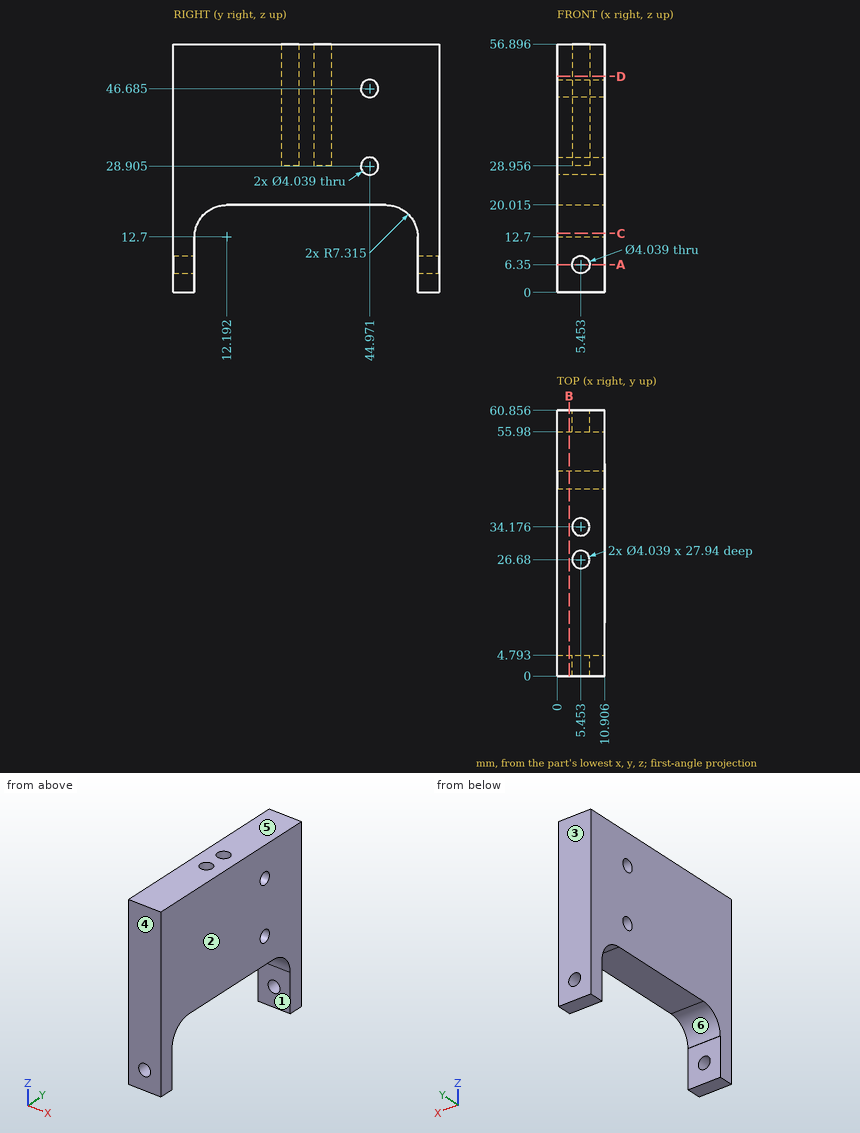
Design review of the part shown in the three views and the two pictorial views. Dimensions are in mm from the part's minimum x, y and z. A direction names the side the tool comes from. Coordinates: 2 decimals unless noted, no trailing zeros. Loops run counter-clockwise (first coordinate to the right, second up) from the corner with the lowest first, then second, coordinate; pieces in that order, holes last.
Q1. We need section D-D on z = 49.5. State the section outline as (x, y) points (1 decimal), and give its area (3 significant figures).
Reported:
outline: (0, 0) - (10.9, 0) - (10.9, 60.9) - (0, 60.9) - close; hole circle Ø4 at (5.5, 26.7); hole circle Ø4 at (5.5, 34.2)
area: 638 mm2
Q2. For pin 1 (3 mm diameter, centred on x = 5.45, y = 26.68, fed in from +Z); pin 2 (2 mm diameter, centred on x = 2, y = 24.5, fed in from -Z) (1 decimal), all flat-tipped, find the tip position at first contact; note any pin that passes through.
Reported:
pin 1: stops at z = 28.96
pin 2: stops at z = 20
Q3. To check wall thickness, follow line 1 (Y direction, x = 3, z = 29) (1 decimal); line 2 (X direction, y = 2.2, z = 6.35) (1 decimal); line 3 (Z direction, x = 6.75, y = 32.5) (1 decimal). State the ranges of each line that lie inside material, in increasing order.
Reported:
line 1: y = 0 to 43, 47 to 60.9
line 2: x = 0 to 3.4, 7.5 to 10.9
line 3: z = 20 to 56.9
Q4. The part is to be moulded in two halves that separate along Y. For the marked faces 3, 4, 5 and 6, say which applies: +Y half, -Y half, draft (parallel to the pull), parting line (faces both ways), or undercut.
Reported:
face 3: +Y half
face 4: -Y half
face 5: draft
face 6: undercut
Q5. We need section A-A on z = 6.35. State the section outline as (x, y) points (1 decimal).
Reported:
outline: (0, 0) - (3.4, 0) - (3.4, 4.8) - (0, 4.8) - close; (0, 56) - (3.4, 56) - (3.4, 60.9) - (0, 60.9) - close; (7.5, 0) - (10.9, 0) - (10.9, 4.8) - (7.5, 4.8) - close; (7.5, 56) - (10.9, 56) - (10.9, 60.9) - (7.5, 60.9) - close
Q6. Tool access review of the marked faces 1 and 2: name each direction out of +Z, -Z, +X, -X, +Y, -Y from which nothing blocks a thin tool from reaching the whole face with its end or side.
Reported:
face 1: -Z, +X, -X
face 2: +Z, -Z, +X, +Y, -Y
Q7. We need section C-C on z = 13.5. State the section outline as (x, y) points (1 decimal), and give its area (3 significant figures).
Reported:
outline: (0, 0) - (10.9, 0) - (10.9, 4.9) - (0, 4.9) - close; (0, 55.9) - (10.9, 55.9) - (10.9, 60.9) - (0, 60.9) - close
area: 107 mm2
Q8. We need section B-B on x = 2.75. State how many separate pieces and enclosed holes the cut face has, and give its area (3 significant figures).
Reported:
separate pieces: 1
enclosed holes: 2
area: 2,440 mm2
